```python
from build123d import *

# Parameters (mm, degrees)
BOSS_EXTRUDE1_DEPTH = 4.3
BOSS_EXTRUDE4_DEPTH = 5.5
FILLET4_R           = 1


with BuildPart() as part:
    # Sketch1 → Boss-Extrude1 (new body)
    with BuildSketch(Plane.XY):
        with BuildLine():
            Line((-2.020725942, -3.5), (-3.211308145, -3.5))
            ThreePointArc((-3.211308145, -3.5), (4.715670166, 0.570048145), (-3.952806323, 2.633974596))
            Line((-3.952806323, 2.633974596), (-2.520725942, 2.633974596))
            Line((-2.520725942, 2.633974596), (-2.020725942, 3.5))
            Line((-2.020725942, 3.5), (2.020725942, 3.5))
            Line((2.020725942, 3.5), (4.041451884, 0))
            Line((4.041451884, 0), (2.020725942, -3.5))
            Line((2.020725942, -3.5), (-2.020725942, -3.5))
        make_face()
        with BuildLine():
            Line((-4.795831523, 4.75), (-3.952806323, 2.633974596))
            ThreePointArc((-3.952806323, 2.633974596), (-2.241776156, 4.18771294), (0, 4.75))
            Line((0, 4.75), (-4.795831523, 4.75))
        make_face()
        with BuildLine():
            Line((-3.211308145, -3.5), (-4.795831523, -4.75))
            Line((-4.795831523, -4.75), (0, -4.75))
            ThreePointArc((0, -4.75), (-1.723006094, -4.426482802), (-3.211308145, -3.5))
        make_face()
    extrude(amount=BOSS_EXTRUDE1_DEPTH)

    # Sketch1<6> → Boss-Extrude4 (add)
    with BuildSketch(Plane.XY):
        with BuildLine():
            ThreePointArc((-4.795831523, -4.75), (6.75, 0), (-4.795831523, 4.75))
            Line((-4.795831523, 4.75), (0, 4.75))
            ThreePointArc((0, 4.75), (4.75, 0), (0, -4.75))
            Line((0, -4.75), (-4.795831523, -4.75))
        make_face()
    extrude(amount=BOSS_EXTRUDE4_DEPTH)

    # Fillet4
    # the kernel refuses this fillet: 1 mm, written as the material it takes off along each edge
    with BuildSketch(Plane(origin=(-4.795831523, -4.75, -3.339360347), x_dir=(0.7851091148875305, 0.6193574716757022, 0), z_dir=(0, 0, 1))) as fillet4_piece_1:
        with BuildLine():
            CenterArc((1.232836015, -1), FILLET4_R, 90, 107.81241463)
            ThreePointArc((0.280772882, -1.305901602), (0.108004206, -0.659913081), (0, 0))
            Line((0, 0), (1.232836015, 0))
        make_face()
    extrude(amount=10.978720693, mode=Mode.SUBTRACT)
    with BuildSketch(Plane(origin=(-3.211308145, -3.5, -0.867394417), x_dir=(1, 0, 0), z_dir=(0, 0, 1))) as fillet4_piece_2:
        with BuildLine():
            CenterArc((FILLET4_R * 0.346957766621, -FILLET4_R), FILLET4_R, 90, 38.269228819)
            Line((-FILLET4_R * 0.272399705055, -FILLET4_R * 0.214890885112), (0, 0))
            Line((0, 0), (FILLET4_R * 0.346957766621, 0))
        make_face()
    extrude(amount=6.034788833, mode=Mode.SUBTRACT)
    with BuildSketch(Plane(origin=(-3.952806323, 2.633974596, -1.695098898), x_dir=(-0.37010921689998283, 0.9289882494228232, 0), z_dir=(0, 0, 1))) as fillet4_piece_3:
        with BuildLine():
            CenterArc((FILLET4_R * 0.678039559156, -FILLET4_R), FILLET4_R, 90, 68.277646872)
            Line((-FILLET4_R * 0.250948690267, -FILLET4_R * 0.6298907831), (0, 0))
            Line((0, 0), (FILLET4_R * 0.678039559156, 0))
        make_face()
    extrude(amount=7.690197796, mode=Mode.SUBTRACT)
    with BuildSketch(Plane(origin=(-4.795831523, 4.75, -1.879489211), x_dir=(0.7421780572784941, 0.6702027538695439, 0), z_dir=(0, 0, 1))) as fillet4_piece_4:
        with BuildLine():
            CenterArc((0.696107115, -0.998448188), FILLET4_R, 86.807628526, 72.832009231)
            Line((-0.241415796, -0.650524644), (0, 0))
            ThreePointArc((0, 0), (0.375897842, 0.010474734), (0.751795684, 0))
        make_face()
    extrude(amount=8.058978421, mode=Mode.SUBTRACT)


solid = part.part
```
Could you check a few things on this model? Use its own coordinates, in mm. A direction names the side the tool comes from. Coordinates: 2 decimals unless noted, no trailing zeros. Write each loop counter-clockwise with the first axis right and the second up, starting at its lowest first coordinate (ties: lowest second). Pieces come first, ordered by that corner, then holes. Notation, with made-up numbers: (74.25, 52.25) -> (120.25, 52.25) arc R25 ccw to (120.25, 80.25) -> close; hole circle Ø10 at (-16.5, 38.5). An arc over 180 degrees is marked (long way). Write item = value, one per line. Start each with the question number.
(1) I want a section at D-D (x = 0.75). Please give me the cut outline in (y, z), plus the area to 3 significant figures.
(2) We'd pull the mould along Y, two halves only. Please class faces 4 (the face through (0, 3.5, 2)), 5 (the face through (4, 2, 0)), 6 (the face through (4.75, 0.1, 4.89)), 7 (the face through (-4.575, 4.738, 2.712)): released by +Y, released by -Y, zero draft, split by the parting line, or undercut.
(3) Will these pins go through, and if not, where does the flat tip stop? pin 1 (1 mm diameter, centred on x = -3.5, z = 5, fed in from -Y); pin 2 (1.3 mm diameter, centred on x = -2.5, z = 5, fed in from +Y); pin 3 (0.8 mm diameter, centred on x = -3, z = 2.5, fed in from -Y).
(4) I want a section at C-C (y = 5.5). Please give me the cut outline in (x, z).
(5) I need wall thicknesses on line 1 (Y direction, x = 3.5, z = 0.5); line 2 (Y direction, x = -2.75, z = 1.25); line 3 (Y direction, x = 6, z = 2.35). Which ranges of each line are inside material? Lowest first, please. Write a range as [from, to].
(6) I want a section at B-B (z = 3.5). Please give me the cut outline in (x, y).
(7) Which directions (+Z, -Z, +X, -X, +Y, -Y) give clear straight access to the entire face, cutting with the end or side of a thin tool? Please do faces 1 (the face through (3, 1.8, 2.1)), 2 (the face through (-3.84, 2.81, 2.12)), 3 (the face through (-2, -4.75, 5)).
(8) I want a section at A-A (x = 3). Please give me the cut outline in (y, z), plus the area to 3 significant figures.
Result set:
q1.outline = (-6.71, 0) -> (-3.5, 0) -> (-3.5, 4.3) -> (-4.69, 4.3) -> (-4.69, 5.5) -> (-6.71, 5.5) -> close; (3.5, 0) -> (6.71, 0) -> (6.71, 5.5) -> (4.69, 5.5) -> (4.69, 4.3) -> (3.5, 4.3) -> close
q1.area = 32.4 mm2
q2.face_4 = undercut
q2.face_5 = zero draft
q2.face_6 = undercut
q2.face_7 = split by the parting line
q3.pin_1 = -6.05
q3.pin_2 = 6.49
q3.pin_3 = -6.23
q4.outline = (-3.91, 0) -> (3.91, 0) -> (3.91, 5.5) -> (-3.91, 5.5) -> close
q5.line_1 = [-5.77, -0.94], [0.94, 5.77]
q5.line_2 = [-6.16, -3.5], [2.63, 6.16]
q5.line_3 = [-3.09, 3.09]
q6.outline = (-4.54, 4.11) -> (-4.2, 3.26) arc R1 ccw to (-3.27, 2.63) -> (-2.52, 2.63) -> (-2.02, 3.5) -> (2.02, 3.5) -> (4.04, 0) -> (2.02, -3.5) -> (-2.86, -3.5) arc R1 ccw to (-3.48, -3.71) -> (-3.83, -3.99) arc R1 ccw to (-3.77, -5.6) arc R6.75 ccw (long way) to (-4.24, 5.25) arc R1 ccw to start
q7.face_1 = +Z, -Z
q7.face_2 = +Z, -Z, -X
q7.face_3 = +Z, -X
q8.outline = (-6.05, 0) -> (-1.8, 0) -> (-1.8, 4.3) -> (-3.68, 4.3) -> (-3.68, 5.5) -> (-6.05, 5.5) -> close; (1.8, 0) -> (6.05, 0) -> (6.05, 5.5) -> (3.68, 5.5) -> (3.68, 4.3) -> (1.8, 4.3) -> close
q8.area = 42.2 mm2
